For this review, take the finished solid that the model builds, in its own axes (mm). Face numbers are marked on the shaded views. A direction names the side the tool comes from. Round coordinates to 2 decimals unless told otherwise and drop trailing zeros. Write each loop counter-clockwise with the first axis right and the second up, starting at its lowest first coordinate (ties: lowest second). Pieces come first, ordered by that corner, then holes. Notation, with made-up numbers: M -23,4 L -2,4 A23 cw -2,25 Z; hole C -20.75,-9 d6. An arc over 180 degrees is marked long. One line per question, with ' | ' between items.
```python
from build123d import *

# Parameters (mm, degrees)
F0_W     = 5.5
F0_H     = 2
F1_DEPTH = 3.5
F2_W     = 4.080000014
F2_H     = 2.080000014
F3_DEPTH = 1.25
F5_DEPTH = 2


with BuildPart() as f1:
    # F0 (on Top) → F1 (new body)
    with BuildSketch(Plane.XY):
        with Locations((1.7311600968, -1.5813936108)):
            Rectangle(F0_W, F0_H)
    extrude(amount=F1_DEPTH)

    # F2 (on face) → F3 (cut, through all)
    with BuildSketch(Plane(origin=(0, -0.5813936108, 0), x_dir=(-1, 0, 0), z_dir=(0, 1, 0))):
        with Locations((-1.7311600968, 1.75)):
            Rectangle(F2_W, F2_H)
    extrude(amount=-F3_DEPTH, mode=Mode.SUBTRACT)

    # F4 (on face) → F5 (join, through all)
    with BuildSketch(Plane(origin=(0, -0.5813936108, 0), x_dir=(-1, 0, 0), z_dir=(0, 1, 0))):
        Polygon((-4.4811600968, 4.5), (-4.4811600968, 3.5), (1.0188399032, 3.5), (9.0188399032, 3.5), (9.0188399032, 4.5), align=None)
    extrude(amount=-F5_DEPTH)

    # F6: F1 across face


with BuildPart() as f1_1:
    add(f1.part)
    add(f1.part.mirror(Plane(origin=(-9.0188399032, -1.5813936108, 4), x_dir=(0, -1, 0), z_dir=(-1, 0, 0))))


solid = f1_1.part
```
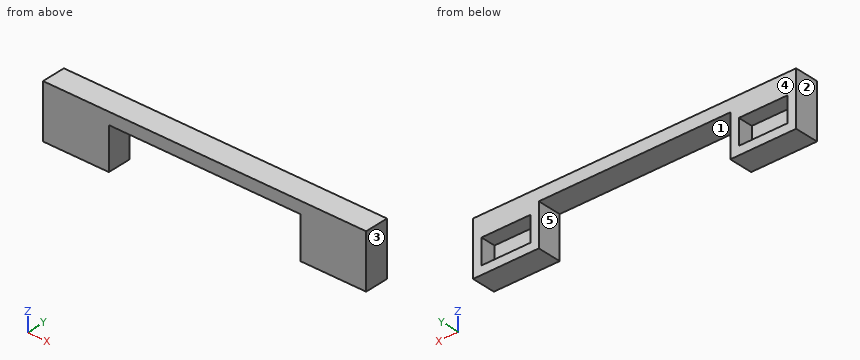
Item 1: Take a section at B-B (x = 1.5). Write out the cut boundary in (y, z).
Results:
outline: M -2.58,0 L -0.58,0 L -0.58,0.71 L -1.83,0.71 L -1.83,2.79 L -0.58,2.79 L -0.58,4.5 L -2.58,4.5 Z
Item 2: Take a section at A-A (z = 3.25). Write out the cut boundary in (x, y).
Results:
outline: M -22.52,-2.58 L -17.02,-2.58 L -17.02,-0.58 L -22.52,-0.58 Z; M -1.02,-2.58 L 4.48,-2.58 L 4.48,-0.58 L -1.02,-0.58 Z
Item 3: Mouldability with a two-part tool opening along X and no side actions: class the marked faces 1, 2 and 3 as +X half, -X half, draft (parallel to the pull), parting line (faces both ways), or undercut.
Results:
face 1: undercut | face 2: -X half | face 3: +X half
Item 4: Insertion check: pin 1 Ø2.5 at (x, z) = (2.5, 1.5) entering from +Y. The pin has a flat end and moves straight along its axis. Give the tip position at first contact, or say it passes through.
Results:
pin 1: y = -0.58
Item 5: To check wall thickness, follow line 1 along X through (y, z) = (-1.3, 2.2); line 2 along X through (y, z) = (-2.3, 2.7); line 3 along Y through (x, z) = (3.5, 2.3). State the ranges of each line that lie inside material, in increasing order. Write a range as from..to.
Results:
line 1: -22.52..-21.81, -17.73..-17.02, -1.02..-0.31, 3.77..4.48 | line 2: -22.52..-17.02, -1.02..4.48 | line 3: -2.58..-1.83
Item 6: Machinability: for the marked faces 4 and 5, which of the approach directions +Z, -Z, +X, -X, +Y, -Y give a long, thin tool a straight path to every point of the face, cutting with its end or side? Answer none if there is none.
Results:
face 4: +Z, -Z, +X, -X, +Y | face 5: -Z, +Y, -Y
Item 7: Take a section at C-C (y = -1.3). Write out the cut boundary in (x, z), then the cut area to 3 significant figures.
Results:
outline: M -22.52,0 L -17.02,0 L -17.02,3.5 L -1.02,3.5 L -1.02,0 L 4.48,0 L 4.48,4.5 L -22.52,4.5 Z; hole M -21.81,0.71 L -17.73,0.71 L -17.73,2.79 L -21.81,2.79 Z; hole M -0.31,0.71 L 3.77,0.71 L 3.77,2.79 L -0.31,2.79 Z | area: 48.5 mm2
Item 8: Take a section at D-D (z = 2.15). Write out the cut boundary in (x, y).
Results:
outline: M -22.52,-2.58 L -17.02,-2.58 L -17.02,-0.58 L -17.73,-0.58 L -17.73,-1.83 L -21.81,-1.83 L -21.81,-0.58 L -22.52,-0.58 Z; M -1.02,-2.58 L 4.48,-2.58 L 4.48,-0.58 L 3.77,-0.58 L 3.77,-1.83 L -0.31,-1.83 L -0.31,-0.58 L -1.02,-0.58 Z
